The model under review builds one solid part; all positions refer to its coordinate system, in mm. Round coordinates to 2 decimals unless told otherwise and drop trailing zeros. Write each loop counter-clockwise with the first axis right and the second up, starting at its lowest first coordinate (ties: lowest second). Pieces come first, ordered by that corner, then holes. Notation, with made-up numbers: M 70,6.5 L 127,6.5 A24 ccw 127,37.5 Z; hole C 13.25,69 d8. An arc over 180 degrees is marked long. One line per item, written item: value. Start each with the question number.
1) Take a section at A-A, the plane y = 13. Write out the cut boundary in (x, z), and give its area (3 significant figures).
2) Take a section at D-D, the plane y = 78. Write out the cut boundary in (x, z).
3) For P1, Ø11, axis at x = -77, y = 13, coming from the +Z side, flat-tipped, find the tip position at first contact; note if it passes through.
4) Take a section at C-C, the plane x = -77. Write out the cut boundary in (y, z), and give its area (3 significant figures).
5) Wall thickness on probe 1 along Y at (x, z) = (-76, 1.85); probe 2 along Y at (x, z) = (-79, 0.3); probe 3 along Y at (x, z) = (-54, 0.65): over which ranges is each line inside the solid? List them lowest first.
6) Take a section at B-B, the plane z = 1.35. Write out the cut boundary in (x, y).
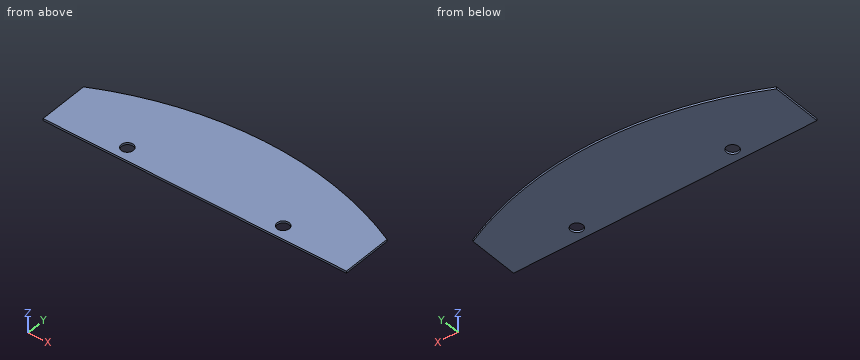
from build123d import *

# Parameters (mm, degrees)
SALIENTE_EXTRUIR1_DEPTH = 2
CROQUIS2_R              = 6
CORTAR_EXTRUIR1_DEPTH   = 173.420996401


with BuildPart() as part:
    # Croquis1 → Saliente-Extruir1 (new body)
    with BuildSketch(Plane.XY):
        with BuildLine():
            Line((-150, 0), (150, 0))
            Line((150, 0), (150, 50))
            ThreePointArc((150, 50), (0, 85), (-150, 50))
            Line((-150, 50), (-150, 0))
        make_face()
    extrude(amount=SALIENTE_EXTRUIR1_DEPTH)

    # Croquis2 → Cortar-Extruir1 (cut, through all)
    with BuildSketch(Plane.XY.offset(2)):
        with Locations((-77, 13)):
            Circle(CROQUIS2_R)
        with Locations((77, 13)):
            Circle(CROQUIS2_R)
    extrude(amount=-CORTAR_EXTRUIR1_DEPTH, mode=Mode.SUBTRACT)


solid = part.part
Checked values:
1. outline: M -150,0 L -83,0 L -83,2 L -150,2 Z; M -71,0 L 71,0 L 71,2 L -71,2 Z; M 83,0 L 150,0 L 150,2 L 83,2 Z
1. area: 552 mm2
2. outline: M -68.53,0 L 68.53,0 L 68.53,2 L -68.53,2 Z
3. P1: passes through
4. outline: M 0,0 L 7,0 L 7,2 L 0,2 Z; M 19,0 L 76.14,0 L 76.14,2 L 19,2 Z
4. area: 128 mm2
5. probe 1: y = 0 to 7.08, 18.92 to 76.37
5. probe 2: y = 0 to 7.34, 18.66 to 75.66
5. probe 3: y = 0 to 80.67
6. outline: M -150,0 L 150,0 L 150,50 A338.93 ccw -150,50 Z; hole C -77,13 d12; hole C 77,13 d12
